```python
from build123d import *

# Parameters (mm, degrees)
SKETCH1_R           = 20
BOSS_EXTRUDE1_DEPTH = 26
CUT_EXTRUDE1_START  = -9
SKETCH3_R           = 20
SKETCH3_R_2         = 5
CUT_EXTRUDE1_DEPTH  = 9
SKETCH4_R           = 1.75
CUT_EXTRUDE2_DEPTH  = 15
CUT_EXTRUDE4_DEPTH  = 2
SKETCH8_R           = 1.5
CUT_EXTRUDE5_DEPTH  = 38.094473982
CUT_EXTRUDE6_START  = -2
SKETCH9_R           = 17.5
SKETCH9_R_2         = 15
SKETCH9_R_3         = 12.5
SKETCH9_R_4         = 10
CUT_EXTRUDE6_DEPTH  = 2
FILLET1_R           = 1
FILLET2_R           = 1
FILLET3_R           = 1
FILLET4_R           = 1
FILLET5_R           = 1
CUT_EXTRUDE7_START  = -1
SKETCH10_R          = 5
CUT_EXTRUDE7_DEPTH  = 1


with BuildPart() as part:
    # Sketch1 → Boss-Extrude1 (new body)
    with BuildSketch(Plane(origin=(0, 0, 0), x_dir=(0, 0, -1), z_dir=(1, 0, 0))):
        with Locations(Location((0, 0, 0), (0, 0, 180))):
            Circle(SKETCH1_R)
    extrude(amount=BOSS_EXTRUDE1_DEPTH)

    # Sketch3 → Cut-Extrude1 (cut)
    with BuildSketch(Plane(origin=(26, 0, 0), x_dir=(0, 0, -1), z_dir=(1, 0, 0)).offset(CUT_EXTRUDE1_START)):
        with Locations(Location((0, 0, 0), (0, 0, 180))):
            Circle(SKETCH3_R)
        Circle(SKETCH3_R_2, mode=Mode.SUBTRACT)
    extrude(amount=CUT_EXTRUDE1_DEPTH, mode=Mode.SUBTRACT)

    # Sketch4 → Cut-Extrude2 (cut)
    with BuildSketch(Plane(origin=(26, 0, 0), x_dir=(0, 0, -1), z_dir=(1, 0, 0))):
        Circle(SKETCH4_R)
    extrude(amount=-CUT_EXTRUDE2_DEPTH, mode=Mode.SUBTRACT)

    # Sketch7 → Cut-Extrude4 (cut)
    with BuildSketch(Plane.ZY):
        with BuildLine():
            Line((-18, 1.5), (-8.518780875, 5.237401303))
            ThreePointArc((-8.518780875, 5.237401303), (-7.147984075, 6.993305632), (-5.422484014, 8.402182283))
            Line((-5.422484014, 8.402182283), (-1.5, 18))
            ThreePointArc((-1.5, 18), (0, 19.5), (1.5, 18))
            Line((1.5, 18), (5.422484014, 8.402182283))
            ThreePointArc((5.422484014, 8.402182283), (7.147984075, 6.993305632), (8.518780875, 5.237401303))
            Line((8.518780875, 5.237401303), (18, 1.5))
            ThreePointArc((18, 1.5), (19.5, 0), (18, -1.5))
            Line((18, -1.5), (8.518780875, -5.237401303))
            ThreePointArc((8.518780875, -5.237401303), (7.147984075, -6.993305632), (5.422484014, -8.402182283))
            Line((5.422484014, -8.402182283), (1.5, -18))
            ThreePointArc((1.5, -18), (0, -19.5), (-1.5, -18))
            Line((-1.5, -18), (-5.422484014, -8.402182283))
            ThreePointArc((-5.422484014, -8.402182283), (-7.147984075, -6.993305632), (-8.518780875, -5.237401303))
            Line((-8.518780875, -5.237401303), (-18, -1.5))
            ThreePointArc((-18, -1.5), (-19.5, 0), (-18, 1.5))
        make_face()
    extrude(amount=-CUT_EXTRUDE4_DEPTH, mode=Mode.SUBTRACT)

    # Sketch8 → Cut-Extrude5 (cut, through all)
    with BuildSketch(Plane.ZY.offset(-2)):
        Circle(SKETCH8_R)
    extrude(amount=-CUT_EXTRUDE5_DEPTH, mode=Mode.SUBTRACT)

    # Sketch9 → Cut-Extrude6 (cut)
    # profile 1 of 2: a face of its own
    with BuildSketch(Plane(origin=(17, 0, 0), x_dir=(0, 0, -1), z_dir=(1, 0, 0)).offset(CUT_EXTRUDE6_START)):
        Circle(SKETCH9_R)
        Circle(SKETCH9_R_2, mode=Mode.SUBTRACT)
    # profile 2 of 2: a face of its own
    with BuildSketch(Plane(origin=(17, 0, 0), x_dir=(0, 0, -1), z_dir=(1, 0, 0)).offset(CUT_EXTRUDE6_START)):
        Circle(SKETCH9_R_3)
        Circle(SKETCH9_R_4, mode=Mode.SUBTRACT)
    extrude(amount=CUT_EXTRUDE6_DEPTH, mode=Mode.SUBTRACT)

    # Fillet1
    fillet1_edges = [part.edges().sort_by_distance(p)[0] for p in [
        (17, 0, 17.5),
    ]]
    fillet(fillet1_edges, radius=FILLET1_R)

    # Fillet2
    fillet2_edges = [part.edges().sort_by_distance(p)[0] for p in [
        (17, 0, -20),
    ]]
    fillet(fillet2_edges, radius=FILLET2_R)

    # Fillet3
    fillet3_edges = [part.edges().sort_by_distance(p)[0] for p in [
        (17, 0, 15),
    ]]
    fillet(fillet3_edges, radius=FILLET3_R)

    # Fillet4
    fillet4_edges = [part.edges().sort_by_distance(p)[0] for p in [
        (17, 0, 12.5),
    ]]
    fillet(fillet4_edges, radius=FILLET4_R)

    # Fillet5
    fillet5_edges = [part.edges().sort_by_distance(p)[0] for p in [
        (17, 0, 10),
    ]]
    fillet(fillet5_edges, radius=FILLET5_R)

    # Sketch10 → Cut-Extrude7 (cut)
    with BuildSketch(Plane(origin=(26, 0, 0), x_dir=(0, 0, -1), z_dir=(1, 0, 0)).offset(CUT_EXTRUDE7_START)):
        Circle(SKETCH10_R)
    extrude(amount=CUT_EXTRUDE7_DEPTH, mode=Mode.SUBTRACT)


solid = part.part
```
Design review of the part built by this model. Coordinates are the model's own, in mm. A direction names the side the tool comes from. Round coordinates to 2 decimals unless told otherwise and drop trailing zeros. Order: outer loops, then holes, each group sorted by start corner. A loop starts at its lowest first (then second) coordinate and runs counter-clockwise, first axis right, second up. Notation, with made-up numbers: (54, 35) - (70, 35) arc R7 cw to (70, 45) - close; hole circle Ø3 at (25, 63). An arc over 180 degrees is marked (long way). Return JSON: item names as keys, results as strings.
Q1. For pin 1 Ø6 at (x, y) = (19, 2) entering from +Z; pin 2 Ø10 at (x, z) = (12.5, 10) entering from +Y; pin 3 Ø12 at (x, z) = (18, -12.5) entering from +Y, all flat-tipped, find the tip position at first contact; note any pin that passes through.
Computed values:
{"pin 1": "stops at z = 19.96", "pin 2": "stops at y = 19.36", "pin 3": "stops at y = 18.8"}
Q2. Wall thickness on L1, parallel to Y at x = 15.2, z = 0; L2, parallel to Y at x = 18.75, z = 0; L3, parallel to Y at x = 4.25, z = 0: over which ranges is each line inside the solid? List them lowest first. Write a range as [from, to].
Computed values:
{"L1": "y = [-20, -17.5], [-15, -12.5], [-10, -1.75], [1.75, 10], [12.5, 15], [17.5, 20]", "L2": "y = [-5, -1.75], [1.75, 5]", "L3": "y = [-20, -1.5], [1.5, 20]"}
Q3. Consider section A-A on x = 2.5. Write out the cut boundary in (y, z).
Computed values:
{"outline": "circle Ø40 at (0, 0); hole circle Ø3 at (0, 0)"}
Q4. Machinability: for faces 5 (the flat face through (25, -2, 0)), 6 (the cylindrical face through (15.493, 3.755, -11.923)), 7 (the flat face through (0.99, 3.34, -13.33)), which of the approach directions +Z, -Z, +X, -X, +Y, -Y give a long, thin tool a straight path to every point of the face, cutting with its end or side? Answer none if there is none.
Computed values:
{"face 5": "+Z, -Z, +X, +Y, -Y", "face 6": "+X", "face 7": "-X"}
Q5. The part is to be moulded in two halves that separate along Z. For faces 1 (the flat face through (0.986, 13.268, 3.434)), 2 (the cylindrical face through (0.99, 6.97, -7.17)), 3 (the cylindrical face through (20.94, -4.88, 1.08)), 4 (the flat face through (0, 9, 9)), say which applies: pulls with the +Z half, pulls with the -Z half, needs draft (parallel to the pull), parting line crosses it, or undercut.
Computed values:
{"face 1": "undercut", "face 2": "undercut", "face 3": "parting line crosses it", "face 4": "needs draft"}
